Autodesk Fusion 360 part; units mm, degrees
sketch "Skizze1" plane through (0, 0, 0) normal (0, 0, 1) x (1, 0, 0)
  line L0 (-18, 20) -> (12, 20)
  line L1 (12, 20) -> (12, -20)
  line L2 (12, -20) -> (-18, -20)
  line L3 (-18, -20) -> (-18, 20)
  line L4 (0, 23) -> (0, -24) construction
  line L5 (-24.4424, 15.24) -> (27, 15.24) construction
  line L6 (-24, -15.24) -> (24, -15.24) construction
  line L7 (-13.79, 18) -> (-13.79, -18.6195) construction
  circle A0 centre (0, 15.24) radius 4.25
  circle A1 centre (0, -15.24) radius 4.25
  circle A2 centre (-13.79, -0.0668) radius 3.5
  circle A3 centre (0, 0) radius 12.25
  line L8 (3.75, -3.75) -> (-3.75, -3.75)
  line L9 (-3.75, -3.75) -> (-3.75, 3.75)
  line L10 (-3.75, 3.75) -> (3.75, 3.75)
  line L11 (3.75, 3.75) -> (3.75, -3.75)
  line L12 (3.75, -3.75) -> (-3.75, 3.75) construction
  line L13 (-3.75, -3.75) -> (3.75, 3.75) construction
  circle A4 centre (0, 0) radius 6.65
  dimension "d1" = 12
  dimension "d2" = 18
  dimension "d3" = 20
  dimension "d4" = 20
  dimension "d5" = 15.24
  dimension "d6" = 15.24
  dimension "d7" = 13.79
  dimension "d8" = 8.5
  dimension "d9" = 8.5
  dimension "d10" = 7
  dimension "d11" = 24.5
  dimension "d12" = 7.5
  dimension "d13" = 7.5
  dimension "d24" = 4.76
  dimension "d25" = 13.3
extrude "Extrusion1" add sketch "Skizze1" along normal blind 8.3 contours L0 L1 L2 L3 A0 A1 A2 A3 | L1 A0 A1 A2 A3 | A0 A3 | A0 A3 | A1 A3 | A1 A3 | A2 A3 | A2 A3 | L8 L9 L10 L11 | A4
extrude "Extrusion6" cut sketch "Skizze1" along normal blind 10 contours A0 A3 | A0 A3 | A1 A3 | A1 A3 | A2 A3 | A2 A3 | L8 L9 L10 L11
extrude "Extrusion7" cut sketch "Skizze1" along normal blind 6.3 contours L1 A0 A1 A2 A3
extrude "Extrusion8" add sketch "Skizze1" against normal blind 1.4 contours A4
The listing builds one solid part. Answer for the finished solid, in the listing's coordinates (mm). A direction names the side the tool comes from. Round coordinates to 2 decimals unless told otherwise and drop trailing zeros. Order: outer loops, then holes, each group sorted by start corner. A loop starts at its lowest first (then second) coordinate and runs counter-clockwise, first axis right, second up. Notation, with made-up numbers: M 58,88 L 81,88 A30 cw 81,122 Z; hole C 88,-14.5 d6. An arc over 180 degrees is marked long. Answer in a Markdown table with one row per item. Add a question column.
1) The part is cut by section A-A on z = 4.25. Determine the outline of the cut face in (x, y).
2) The part is cut by section C-C on y = -15.24. Determine the outline of the cut face in (x, z).
3) Consider line 1 along Y through (x, z) = (0, 4.75); line 2 along X through (y, z) = (15, 6.25); line 3 along Y through (x, z) = (-1, 7). Determine where each line is inside the solid, lowest interval first. Write a range as from..to.
4) The part is cut by section D-D on x = 0. Determine the outline of the cut face in (y, z).
5) Determine the mould class of faces 1 (the face through (4, 0, -1.4)), 2 (the face through (-0.92, 19.39, 4.09)), 3 (the face through (-0.553, -19.454, 4.092)), 4 (the face through (-18, 0, 4)) for opening direction X: pulls with the +X half, pulls with the -X half, needs draft (parallel to the pull), parting line crosses it, or undercut.
6) Which of the six approach directions +Z, -Z, +X, -X, +Y, -Y give full straight-line access (tool end or side, diameter ignored) to faces 5 (the face through (-8.66, 8.664, 3.106)), 6 (the face through (0, 3.75, 4)), 7 (the face through (12, 0, 7))?
7) The part is cut by section B-B on x = -13.79. Determine the outline of the cut face in (y, z).
Findings below:
| question | item | result |
|---|---|---|
| 1 | outline | M -18,-20 L 12,-20 L 12,-2.46 A12.25 cw 2.69,-11.95 A4.25 cw long -2.69,-11.95 A12.25 cw -11.88,-3 A3.5 cw long -11.91,2.88 A12.25 cw -2.69,11.95 A4.25 cw long 2.69,11.95 A12.25 cw 12,2.46 L 12,20 L -18,20 Z; C 0,0 d13.3; hole M -3.75,-3.75 L 3.75,-3.75 L 3.75,3.75 L -3.75,3.75 Z |
| 2 | outline | M -18,0 L -4.25,0 L -4.25,8.3 L -18,8.3 Z; M 4.25,0 L 12,0 L 12,8.3 L 4.25,8.3 Z |
| 3 | line 1 | y = -20..-19.49, -6.65..-3.75, 3.75..6.65, 19.49..20 |
| 3 | line 2 | x = -18..-4.24, 4.24..12 |
| 3 | line 3 | y = -20..-19.37, -11.11..-3.75, 3.75..11.11, 19.37..20 |
| 4 | outline | M -20,0 L -19.49,0 L -19.49,8.3 L -20,8.3 Z; M -10.99,6.3 L -6.65,6.3 L -6.65,-1.4 L -3.75,-1.4 L -3.75,8.3 L -10.99,8.3 Z; M 3.75,-1.4 L 6.65,-1.4 L 6.65,6.3 L 10.99,6.3 L 10.99,8.3 L 3.75,8.3 Z; M 19.49,0 L 20,0 L 20,8.3 L 19.49,8.3 Z |
| 5 | face 1 | needs draft |
| 5 | face 2 | undercut |
| 5 | face 3 | undercut |
| 5 | face 4 | pulls with the -X half |
| 6 | face 5 | -Z |
| 6 | face 6 | +Z, -Z |
| 6 | face 7 | +Z, -Z, +X, +Y, -Y |
| 7 | outline | M -20,0 L -3.57,0 L -3.57,8.3 L -20,8.3 Z; M 3.43,0 L 20,0 L 20,8.3 L 3.43,8.3 Z |
